Autodesk Inventor part; units mm, degrees
ref_plane "Start Plane" through (0, 0, 100) normal (0, 0, 1) x (1, 0, 0)
ref_plane "End Plane" through (0, 0, 726.1299) normal (0, 0, 1) x (1, 0, 0)
ref_plane "Work Plane4" through (696.1299, -24, 0) normal (0.7071, 0, 0.7071) x (0.7071, 0, -0.7071)
ref_plane "Start Plane" through (0, 0, 100) normal (0, 0, 1) x (1, 0, 0)
ref_plane "End Plane" through (0, 0, 726.1299) normal (0, 0, 1) x (1, 0, 0)
sketch "Sketch" plane through (0, 0, 0) normal (0, 0, 1) x (1, 0, 0)
  line L0 (-30, -24) -> (-30, 24)
  line L1 (-24, 30) -> (24, 30)
  line L2 (30, 24) -> (30, -24)
  line L3 (24, -30) -> (-24, -30)
  arc A0 (-30, -24) -> (-24, -30) centre (-24, -24) ccw
  arc A1 (30, 24) -> (24, 30) centre (24, 24) ccw
  arc A2 (-24, 30) -> (-30, 24) centre (-24, 24) ccw
  arc A3 (24, -30) -> (30, -24) centre (24, -24) ccw
  arc A4 (-24, 27) -> (-27, 24) centre (-24, 24) ccw
  line L4 (-24, 27) -> (24, 27)
  arc A5 (27, 24) -> (24, 27) centre (24, 24) ccw
  line L5 (27, 24) -> (27, -24)
  arc A6 (24, -27) -> (27, -24) centre (24, -24) ccw
  line L6 (24, -27) -> (-24, -27)
  arc A7 (-27, -24) -> (-24, -27) centre (-24, -24) ccw
  line L7 (-27, -24) -> (-27, 24)
  line L8 (0, 43.7397) -> (0, -43.7397) construction
  line L9 (-43.7397, 0) -> (43.7397, 0) construction
  dimension "d7" = 6
  dimension "d9" = 60
  dimension "d11" = 60
  dimension "d12" = 3
  dimension "d15" = 30
  dimension "d16" = 30
extrude "Body" add sketch "Sketch" along normal up to surface (626.1299 mm away) from surface at 100
sketch "Sketch3" plane through (0, 0, 0) normal (0, 0, 1) x (1, 0, 0)
  line L0 (0, 0) -> (10, 0)
ref_plane "Work Plane3" through (0, 0, 0) normal (0, -1, 0) x (1, 0, 0)
ref_plane "Work Plane4" through (696.1299, -24, 0) normal (0.7071, 0, 0.7071) x (0.7071, 0, -0.7071)
split "Split1" plane through (696.1299, -24, 0) removes the side toward (0.7071, 0, 0.7071)
sketch "Sketch4" plane through (0, 0, 0) normal (0, -1, 0) x (1, 0, 0)
  line L0 (-2, 100) -> (12, 100)
  line L1 (-2, 726.1299) -> (12, 726.1299)
  dimension "d18" = 626.1299
equation "\"d7\" = G_IR"
equation "\"d9\" = G_W"
equation "\"d11\" = G_H"
equation "\"d12\" = G_T"
equation "\"d15\" = 0.5 * d9"
equation "\"d16\" = 0.5 * d11"
equation "\"d3\" = G_L"
equation "\"G_W\" = 60"
equation "\"G_H\" = 60"
equation "\"G_T\" = 3"
equation "\"G_IR\" = 6"
equation "\"G_L\" = d18"
equation "\"G_OFFSET_END\" = 0"
equation "\"d14\" = G_OFFSET_END + B_L"
equation "\"B_L\" = 726.12992"
properties part number "ISO 10799-2 - 60x60x3 - 626,13" material "Steel, Mild"
The model under review builds one solid part; all positions refer to its coordinate system, in mm. A direction names the side the tool comes from. Coordinates: 2 decimals unless noted, no trailing zeros. Write each loop counter-clockwise with the first axis right and the second up, starting at its lowest first coordinate (ties: lowest second). Pieces come first, ordered by that corner, then holes. Notation, with made-up numbers: M 23,3.5 L 78,3.5 A18 cw 78,17.5 Z; hole C -11,13 d6. An arc over 180 degrees is marked long. Put each result on its own line as item: value.
1) Wall thickness on probe 1 along Y at (x, z) = (0.5, 571); probe 2 along Y at (x, z) = (26, 207.5): over which ranges is each line inside the solid? List them lowest first. Write a range as [from, to].
Computed:
probe 1: y = [-30, -27], [27, 30]
probe 2: y = [-29.66, -26.24], [26.24, 29.66]
2) Add section A-A on z = 492. Give the boundary of the cut face in (x, y).
Computed:
outline: M -30,-24 A6 ccw -24,-30 L 24,-30 A6 ccw 30,-24 L 30,24 A6 ccw 24,30 L -24,30 A6 ccw -30,24 Z; hole M -27,-24 A3 ccw -24,-27 L 24,-27 A3 ccw 27,-24 L 27,24 A3 ccw 24,27 L -24,27 A3 ccw -27,24 Z
3) Add section B-B on y = -10. Give the boundary of the cut face in (x, z), then the cut area to 3 significant figures.
Computed:
outline: M -30,100 L -27,100 L -27,723.13 L -30,726.13 Z; M 27,100 L 30,100 L 30,666.13 L 27,669.13 Z
area: 3,580 mm2
4) Draft analysis for pull direction Y (two halves, no side actions). For faces 3 (the flat face through (0, 30, 406)), 4 (the flat face through (-2, -29, 100)), 5 (the flat face through (-27, 0, 407)), 6 (the flat face through (0, -27, 406)), state which applies: released by +Y, released by -Y, zero draft, split by the parting line, or undercut.
Computed:
face 3: released by +Y
face 4: zero draft
face 5: undercut
face 6: undercut
5) Add section C-C on x = -17. Give the boundary of the cut face in (y, z).
Computed:
outline: M -30,100 L -27,100 L -27,713.13 L -30,713.13 Z; M 27,100 L 30,100 L 30,713.13 L 27,713.13 Z
6) For faces 1 (the flat face through (27, 0, 381)), 2 (the flat face through (0, -30, 406)), list the 3-axis set-ups (+Z, -Z, +X, -X, +Y, -Y) from which the entire face can be reached by the end or side of a thin tool; tool diameter is ignored.
Computed:
face 1: +Z, -Z
face 2: +Z, -Z, +X, -X, -Y
